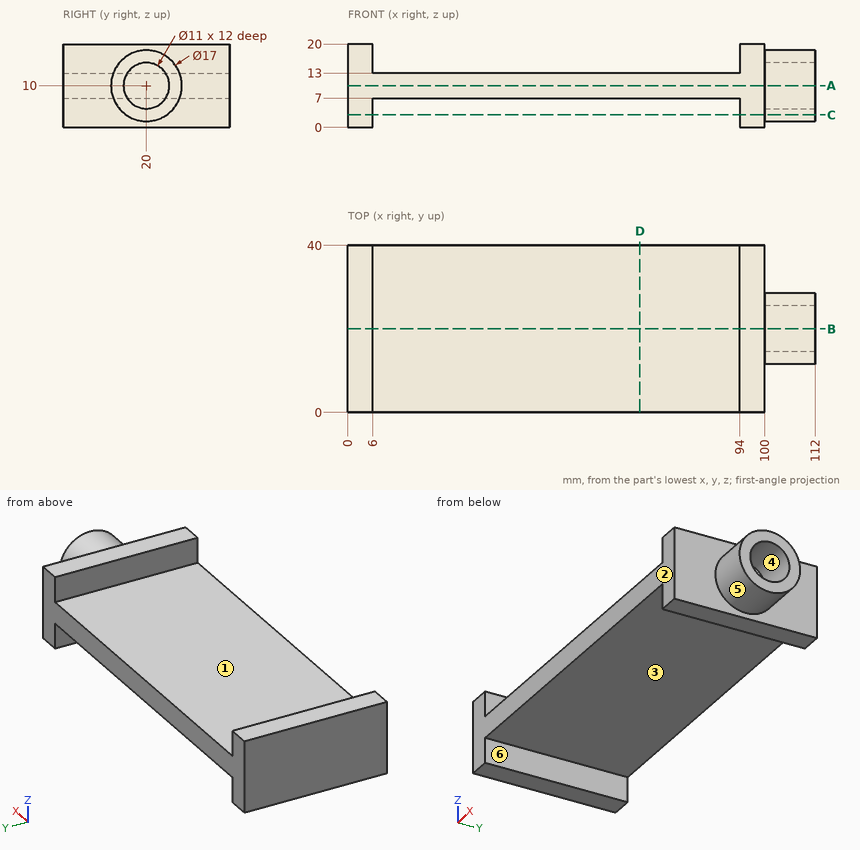
Source: three-view drawing plus pictorial views. Frame: mm from the lowest corner of the part. A direction names the side the tool comes from. Round coordinates to 2 decimals unless told otherwise and drop trailing zeros. Write each loop counter-clockwise with the first axis right and the second up, starting at its lowest first coordinate (ties: lowest second). Pieces come first, ordered by that corner, then holes. Notation, with made-up numbers: M 7,41 L 14,41 A28 ccw 14,63 Z; hole C -18,20.25 d11. An arc over 180 degrees is marked long. Use CSV: the item, a comma, the result in double quotes. Start each with the question number.
Q1. Pull-direction query (Y, two-part tool) for the marked faces 4, 5 and 6; classes: +Y half, -Y half, draft (parallel to the pull), parting line (faces both ways), or undercut.
Q2. Cut plane D-D on x = 70. Output: boundary loops of the cut face in (y, z), plus the area to 3 significant figures.
Q3. Access query for the marked faces 1, 2 and 3. Directions: +Z, -Z, +X, -X, +Y, -Y. A direction counts if a zero-diameter tool reaches every point of the face in a straight line with its end or side. Return the directions, or none.
Q4. Cut plane A-A on z = 10. Output: boundary loops of the cut face in (x, y).
Q5. Cut plane C-C on z = 3. Output: boundary loops of the cut face in (x, y).
Q6. Line query: line 1 (X direction, y = 2, z = 17.5); line 2 (Y direction, x = 108.5, z = 10); line 3 (X direction, y = 15, z = 13.75). Output: solid intervals per line, ascending. Write a range as from..to.
Q7. First-contact query: P1, Ø2, axis at y = 30, z = 15.5, coming from the +X side; P2, Ø10, axis at x = 28.5, y = 36, coming from the +Z side. Flat tips, straight axial feed; report the tip coordinate or a pass-through.
Q8. Cut plane B-B on y = 20. Output: boundary loops of the cut face in (x, z).
Results found:
1,face 4,"undercut"
1,face 5,"parting line"
1,face 6,"draft"
2,outline,"M 0,7 L 40,7 L 40,13 L 0,13 Z"
2,area,"240 mm^2"
3,face 1,"+Z, +Y, -Y"
3,face 2,"+Z, -Z, +X, -X, -Y"
3,face 3,"-Z, +Y, -Y"
4,outline,"M 0,0 L 100,0 L 100,11.5 L 112,11.5 L 112,14.5 L 100,14.5 L 100,25.5 L 112,25.5 L 112,28.5 L 100,28.5 L 100,40 L 0,40 Z"
5,outline,"M 0,0 L 6,0 L 6,40 L 0,40 Z; M 94,0 L 100,0 L 100,15.18 L 112,15.18 L 112,24.82 L 100,24.82 L 100,40 L 94,40 Z"
6,line 1,"0..6, 94..100"
6,line 2,"11.5..14.5, 25.5..28.5"
6,line 3,"0..6, 94..112"
7,P1,"x = 100"
7,P2,"z = 13"
8,outline,"M 0,0 L 6,0 L 6,7 L 94,7 L 94,0 L 100,0 L 100,1.5 L 112,1.5 L 112,4.5 L 100,4.5 L 100,15.5 L 112,15.5 L 112,18.5 L 100,18.5 L 100,20 L 94,20 L 94,13 L 6,13 L 6,20 L 0,20 Z"
